```python
from build123d import *

# Parameters (mm, degrees)
F0_R      = 1.7
F0_W      = 23.3248192817
F0_H      = 35.4459092319
F0_H_2    = 20
F1_DEPTH  = 5
F2_R      = 3
F2_R_2    = 1.7
F3_DEPTH  = 4
F4_W      = 15
F4_H      = 15
F5_DEPTH  = 25
F6_R      = 5
F7_DEPTH  = 15
F8_R      = 2
F9_R      = 1.875
F10_DEPTH = 7
F11_R     = 5


with BuildPart() as f1:
    # F0 (on Top) → F1 (new body)
    with BuildSketch(Plane.XY):
        Polygon((23.3248192817, 0), (0, 0), (0, -7), (23.3248192817, -7), (37, -7), (37, 0), align=None)
        with Locations((3.5, -3.5)):
            Circle(F0_R, mode=Mode.SUBTRACT)
        with Locations((33.5, -3.5)):
            Circle(F0_R, mode=Mode.SUBTRACT)
        with Locations((11.6624096408, -24.722954616)):
            Rectangle(F0_W, F0_H)
        with Locations((11.6624096408, 10)):
            Rectangle(F0_W, F0_H_2)
        with BuildLine():
            Line((0, -7), (0, 0))
            Line((0, 0), (0, 20))
            Line((0, 20), (-4.9525605589, 20))
            Line((-4.9525605589, 20), (-4.9525605589, -9.2811752111))
            ThreePointArc((-4.9525605589, -9.2811752111), (-8.9525605589, -13.2811752111), (-12.9525605589, -9.2811752111))
            Line((-12.9525605589, -9.2811752111), (-12.9525605589, 20))
            Line((-12.9525605589, 20), (-18.2450078428, 20))
            Line((-18.2450078428, 20), (-18.2450078428, -42.4459092319))
            Line((-18.2450078428, -42.4459092319), (0, -42.4459092319))
            Line((0, -42.4459092319), (0, -7))
        make_face()
    extrude(amount=F1_DEPTH)

    # F2 (on face) → F3 (cut)
    with BuildSketch(Plane.XY.offset(5)):
        with Locations((3.5, -3.5)):
            Circle(F2_R)
        with Locations((3.5, -3.5)):
            Circle(F2_R_2, mode=Mode.SUBTRACT)
        with Locations((33.5, -3.5)):
            Circle(F2_R)
        with Locations((33.5, -3.5)):
            Circle(F2_R_2, mode=Mode.SUBTRACT)
    extrude(amount=-F3_DEPTH, mode=Mode.SUBTRACT)

    # F4 (on face) → F5 (join)
    with BuildSketch(Plane.XY.offset(5)):
        with Locations((-8.9525605589, -32.2227959335)):
            Rectangle(F4_W, F4_H)
    extrude(amount=F5_DEPTH)

    # F6 (on face) → F7 (cut)
    with BuildSketch(Plane(origin=(0, -24.7227959335, 0), x_dir=(-1, 0, 0), z_dir=(0, 1, 0))):
        with Locations((8.9525605589, 20)):
            Circle(F6_R)
    extrude(amount=-F7_DEPTH, mode=Mode.SUBTRACT)

    # F8
    f8_edges = [f1.edges().sort_by_distance(p)[0] for p in [
        (23.324819, 20, 2.5),
        (37, 0, 2.5),
        (37, -7, 2.5),
        (23.324819, -42.445909, 2.5),
        (-18.245008, 20, 2.5),
        (-18.245008, -42.445909, 2.5),
        (23.324819, -7, 2.5),
        (-4.952561, 20, 2.5),
        (-12.952561, 20, 2.5),
    ]]
    fillet(f8_edges, radius=F8_R)

    # F9 (on face) → F10 (cut)
    with BuildSketch(Plane.XY.offset(30)):
        with Locations((-8.9525605589, -32.2227959335)):
            Circle(F9_R)
    extrude(amount=-F10_DEPTH, mode=Mode.SUBTRACT)

    # F11
    f11_edges = [f1.edges().sort_by_distance(p)[0] for p in [
        (-1.452561, -32.222796, 30),
        (-16.452561, -32.222796, 30),
    ]]
    fillet(f11_edges, radius=F11_R)


solid = f1.part
```
Here's how the part is built. I have some questions about the finished solid (model axes, mm). A direction names the side the tool comes from. Round coordinates to 2 decimals unless told otherwise and drop trailing zeros. Order: outer loops, then holes, each group sorted by start corner. A loop starts at its lowest first (then second) coordinate and runs counter-clockwise, first axis right, second up. Notation, with made-up numbers: (-5, 55) -> (31, 55) arc R32 cw to (31, 91) -> close; hole circle Ø5 at (3.25, -38.75). An arc over 180 degrees is marked (long way). Use a Markdown table: item, result. Add a question column.
(1) For pin 1 Ø12 at (y, z) = (-14, 8) entering from +X; pin 2 Ø6 at (x, y) = (20.5, -29.5) entering from +Z; pin 3 Ø6 at (x, y) = (-8.95, -32.22) entering from +Z; pin 4 Ø1.5 at (x, z) = (27.5, 3) entering from +Y, each with a flat end and sliding along its axis, tell me the tip position at first contact or that it passes through.
(2) I need wall thicknesses on line 1 along Y through (x, z) = (33.5, 0.55); line 2 along X through (y, z) = (-6, 4) (3 decimals); line 3 along Y through (x, z) = (-7, 6). Which ranges of each line are inside material? Lowest first, please.
(3) Suppose I cut it at A-A, the plane x = 3.5. Please give me the cut outline in (y, z), and give its area (3 significant figures).
(4) Suppose I cut it at B-B, the plane y = -3.5. Please give me the cut outline in (x, z) (3 decimals).
(5) Suppose I cut it at D-D, the plane x = 33.5. Please give me the cut outline in (y, z), and give its area (3 significant figures).
(6) Suppose I cut it at C-C, the plane z = 20. Please give me the cut outline in (x, y).
(7) If we mould it in two halves opening along Y, with no side actions, what happens to faces 6 (the face through (5, -5, 1)), 7 (the face through (0.5, -3.4, 3)), 8 (the face through (-4.35, 19.43, 2.54)), 9 (the face through (-4.953, 5, 2))? For each: released by +Y, released by -Y, zero draft, split by the parting line, or undercut.
(8) For faces 1 (the face through (30.5, -3.4, 3)), 2 (the face through (-12.953, 4, 2)), 3 (the face through (-9.1, -39.723, 14.5)), 4 (the face through (-16.453, -32, 15)), 5 (the face through (-9.1, -24.723, 14.5)), which set-ups out of +Z, -Z, +X, -X, +Y, -Y let a thin tool reach every point of the face, with its end or its side?
Verdict:
| question | item | result |
|---|---|---|
| 1 | pin 1 | x = 23.33 |
| 1 | pin 2 | z = 5 |
| 1 | pin 3 | z = 30 |
| 1 | pin 4 | y = 0 |
| 2 | line 1 | -7 to -5.2, -1.8 to 0 |
| 2 | line 2 | -18.245 to -12.953, -4.953 to 1.842, 5.158 to 31.842, 35.158 to 36.732 |
| 2 | line 3 | -39.72 to -24.72 |
| 3 | outline | (-42.45, 0) -> (-5.2, 0) -> (-5.2, 1) -> (-6.5, 1) -> (-6.5, 5) -> (-42.45, 5) -> close; (-1.8, 0) -> (20, 0) -> (20, 5) -> (-0.5, 5) -> (-0.5, 1) -> (-1.8, 1) -> close |
| 3 | area | 285 mm2 |
| 4 | outline | (-18.245, 0) -> (-12.953, 0) -> (-12.953, 5) -> (-18.245, 5) -> close; (-4.953, 0) -> (1.8, 0) -> (1.8, 1) -> (0.5, 1) -> (0.5, 5) -> (-4.953, 5) -> close; (5.2, 0) -> (31.8, 0) -> (31.8, 1) -> (30.5, 1) -> (30.5, 5) -> (6.5, 5) -> (6.5, 1) -> (5.2, 1) -> close; (35.2, 0) -> (37, 0) -> (37, 5) -> (36.5, 5) -> (36.5, 1) -> (35.2, 1) -> close |
| 5 | outline | (-7, 0) -> (-5.2, 0) -> (-5.2, 1) -> (-6.5, 1) -> (-6.5, 5) -> (-7, 5) -> close; (-1.8, 0) -> (0, 0) -> (0, 5) -> (-0.5, 5) -> (-0.5, 1) -> (-1.8, 1) -> close |
| 5 | area | 7.60 mm2 |
| 6 | outline | (-16.45, -39.72) -> (-13.95, -39.72) -> (-13.95, -24.72) -> (-16.45, -24.72) -> close; (-3.95, -39.72) -> (-1.45, -39.72) -> (-1.45, -24.72) -> (-3.95, -24.72) -> close |
| 7 | face 6 | undercut |
| 7 | face 7 | undercut |
| 7 | face 8 | released by +Y |
| 7 | face 9 | zero draft |
| 8 | face 1 | +Z |
| 8 | face 2 | +Z, -Z, +Y |
| 8 | face 3 | +Z, +X, -X, -Y |
| 8 | face 4 | +Z, -X, +Y, -Y |
| 8 | face 5 | +Z, +X, -X, +Y |
